Here's how the part is built. I have some questions about the finished solid (model axes, mm). A direction names the side the tool comes from. Round coordinates to 2 decimals unless told otherwise and drop trailing zeros. Write each loop counter-clockwise with the first axis right and the second up, starting at its lowest first coordinate (ties: lowest second). Pieces come first, ordered by that corner, then holes. Notation, with made-up numbers: M 45,46 L 99,46 A24 cw 99,73 Z; hole C 21.25,63 d3. An arc over 180 degrees is marked long. Use one line per item in the form item = value. Start each with the question number.
Q1. I'm going to push flat-ended pins straight in: pin 1 Ø5 at (x, z) = (-75, 10.5) entering from +Y; pin 2 Ø1.5 at (x, y) = (-59, -130) entering from +Z; pin 3 Ø17 at (x, z) = (-62.33, 16.15) entering from +Y; pin 4 Ø2 at (x, z) = (-50.5, 63) entering from +Y. Where does each tip first touch, or does it pass through?
Q2. I need wall thicknesses on line 1 along X through (y, z) = (-207.5, 25); line 2 along Z through (x, y) = (-66.5, -34.5); line 3 along Y through (x, z) = (-66.5, 26). Which ranges of each line are inside material? Lowest first, please. Write a range as from..to.
Q3. I want a section at B-B on y = -82. List the corners of the cut face in (x, z) for me, and give its area (3 significant figures).
Q4. I want a section at A-A on z = 47. List the corners of the cut face in (x, y) for me, and give its area (3 significant figures).
Q5. We'd pull the mould along X, two halves only. Please class faces 3 (the face through (-40.577, -47.542, 46.256)), 4 (the face through (-63, -124, 3)), 5 (the face through (-79.1, -23.63, 49.95)), 6 (the face through (-38.564, -150.441, 2.284)): +X half, -X half, draft (parallel to the pull), parting line (faces both ways), or undercut.
Q6. For faces 1 (the face through (-62, -247, 46)), 2 (the face through (-85.444, -245.86, 49.954)), which set-ups out of +Z, -Z, +X, -X, +Y, -Y let a thin tool reach every point of the face, with its end or its side?
Autodesk Fusion 360 part; units mm, degrees
sketch "Sketch1" plane through (0, 0, 0) normal (0, 0, 1) x (1, 0, 0)
  line L0 (-36.1553, -250) -> (-89.3702, -250)
  line L1 (-89.3702, -250) -> (-89.3702, 17.3508)
  line L2 (-89.3702, 17.3508) -> (-36.1553, 17.3508)
  line L3 (-36.1553, 17.3508) -> (-36.1553, -250)
extrude "Extrude1" add sketch "Sketch1" along normal blind 90.7403
sketch "Sketch2" plane through (0, 0, 90.7403) normal (0, 0, 1) x (-1, 0, 0)
  line L0 (36.1553, -17.3508) -> (89.3702, -17.3508)
  line L1 (89.3702, -17.3508) -> (89.3702, 250)
  line L2 (89.3702, 250) -> (36.1553, 250)
  line L3 (36.1553, 250) -> (36.1553, -17.3508)
  line L4 (89.3702, 49.3912) -> (62.7627, -17.3508)
  line L5 (62.7627, -17.3508) -> (36.1553, 46.8639)
extrude "Extrude2" cut sketch "Sketch2" against normal blind 218.776 contours L0 L3 L5 | L0 L1 L4
fillet "Fillet1" radius 11.437 1 edges at (-62.7627, 17.3508, 45.3701)
fillet "Fillet2" radius 63.498 1 edges at (-89.3702, -49.3912, 45.3701)
fillet "Fillet3" radius 74.946 1 edges at (-36.1553, -46.8639, 45.3701)
fillet "Fillet4" radius 13.769 1 edges at (-89.3702, -250, 45.3701)
fillet "Fillet5" radius 13.342 1 edges at (-36.1553, -250, 45.3701)
shell "Shell1" thickness 3 removed faces 1 at (-53.8936, -178.2217, 90.7403)
fillet "Fillet8" radius 8.009 1 faces at (-53.8936, -178.2217, 0)
hole "Hole2" at (-62.3327, -250, 16.1469) direction (0, 1, 0) diameter 21 depth 30 tip angle 118
Reported:
q1.pin_1 = -7.37
q1.pin_2 = 3
q1.pin_3 = -1.58
q1.pin_4 = -9.83
q2.line_1 = -89.37..-86.37, -39.16..-36.16
q2.line_2 = 0..3
q2.line_3 = -250..-247, -5.56..-2.28
q3.outline = M -89.37,8.01 A8.01 ccw -81.36,0 L -44.16,0 A8.01 ccw -36.16,8.01 L -36.16,90.74 L -39.16,90.74 L -39.16,3 L -86.37,3 L -86.37,90.74 L -89.37,90.74 Z
q3.area = 659 mm^2
q4.outline = M -89.37,-236.23 A13.77 ccw -75.6,-250 L -49.5,-250 A13.34 ccw -36.16,-236.66 L -36.16,-61.78 A74.95 ccw -41.86,-33.09 L -51.99,-8.64 A11.44 ccw -73.18,-8.79 L -84.86,-38.07 A63.5 ccw -89.37,-61.58 Z; hole M -86.37,-236.23 A10.77 ccw -75.6,-247 L -49.5,-247 A10.34 ccw -39.16,-236.66 L -39.16,-61.78 A71.95 ccw -44.64,-34.24 L -54.76,-9.79 A8.44 ccw -70.4,-9.9 L -82.07,-39.18 A60.5 ccw -86.37,-61.58 Z
q4.area = 1,640 mm^2
q5.face_3 = undercut
q5.face_4 = undercut
q5.face_5 = -X half
q5.face_6 = +X half
q6.face_1 = +Z
q6.face_2 = +Z, -Z, -X, -Y
